For this review, take the finished solid that the model builds, in its own axes (mm). Face numbers are marked on the shaded views. A direction names the side the tool comes from. Coordinates: 2 decimals unless noted, no trailing zeros. Loops run counter-clockwise (first coordinate to the right, second up) from the corner with the lowest first, then second, coordinate; pieces in that order, holes last. Notation, with made-up numbers: (62.5, 39.5) -> (118.5, 39.5) arc R19 cw to (118.5, 43.5) -> close; hole circle Ø5 at (61.25, 77). An arc over 180 degrees is marked (long way). One line per item, written item: value.
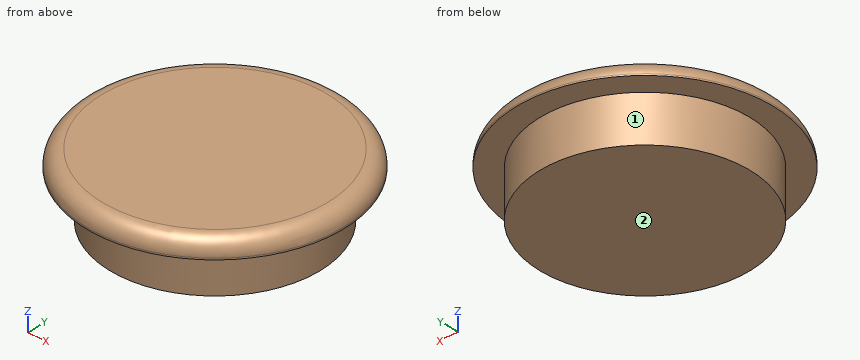
Autodesk Fusion 360 part; units mm, degrees
sketch "Sketch1" plane through (0, 0, 0) normal (0, 0, 1) x (1, 0, 0)
  circle A0 centre (0, 0) radius 13.5
  circle A1 centre (0, 0) radius 16.5
  dimension "d1" = 27
  dimension "d2" = 33
extrude "Extrude1" add sketch "Sketch1" along normal blind 2.2 contours A0 | A1
extrude "Extrude2" add sketch "Sketch1" against normal blind 6 contours A0
fillet "Fillet1" radius 2 1 edges at (-15.3834, -5.9667, 2.2)
1. For the marked faces 1 and 2, list the 3-axis set-ups (+Z, -Z, +X, -X, +Y, -Y) from which the entire face can be reached by the end or side of a thin tool; tool diameter is ignored.
Return value:
face 1: -Z
face 2: -Z, +X, -X, +Y, -Y
2. To check wall thickness, follow probe 1 along Z at (x, y) = (13.5, -2); probe 2 along Y at (x, z) = (9, -0.5); probe 3 along X at (y, z) = (12.5, -2). State the ranges of each line that lie inside material, in increasing order. Write a range as from..to.
Return value:
probe 1: z = 0..2.2
probe 2: y = -10.06..10.06
probe 3: x = -5.1..5.1
3. Take a section at C-C, the plane z = -1.5. Give the boundary of the cut face in (x, y), and give its area (3 significant figures).
Return value:
outline: circle Ø27 at (0, 0)
area: 573 mm2
4. Insertion check: pin 1 Ø1.5 at (x, z) = (-6, 0) entering from +Y; pin 2 Ø2 at (y, z) = (-1.5, -1.5) entering from +X; pin 3 Ø3 at (y, z) = (-3.5, -3.5) entering from +X. Each pin has a flat end and moves straight along its axis. Give the tip position at first contact, or say it passes through.
Return value:
pin 1: stops at y = 15.64
pin 2: stops at x = 13.49
pin 3: stops at x = 13.35
5. Take a section at A-A, the plane y = 0. Give the boundary of the cut face in (x, z).
Return value:
outline: (-16.5, 0) -> (-13.5, 0) -> (-13.5, -6) -> (13.5, -6) -> (13.5, 0) -> (16.5, 0) -> (16.5, 0.2) arc R2 ccw to (14.5, 2.2) -> (-14.5, 2.2) arc R2 ccw to (-16.5, 0.2) -> close
